Verification items for the finished model (mm, model axes). Face numbers are marked on the shaded views. A direction names the side the tool comes from. Round coordinates to 2 decimals unless told otherwise and drop trailing zeros. Write each loop counter-clockwise with the first axis right and the second up, starting at its lowest first coordinate (ties: lowest second). Pieces come first, ordered by that corner, then holes. Notation, with made-up numbers: (-29.75, 43.25) - (-23.75, 43.25) arc R33 ccw to (-23.75, 73.25) - close; hole circle Ø4 at (-13, 31.25). An arc over 180 degrees is marked (long way). Answer as a JSON object with one key per item and string values.
```python
from build123d import *

# Parameters (mm, degrees)
SCHIZZO2_R               = 4.5
TAGLIO_ESTRUSIONE1_DEPTH = 60.933296255


with BuildPart() as part:
    # Schizzo1 → Rivoluzione1 (revolve)
    with BuildSketch(Plane.XY):
        Polygon((0, 0), (0, 42), (5, 42), (5, 26), (7.5, 26), (7.5, 23.25), (11, 23.25), (11, 26), (13, 26), (13, 20), (5, 20), (5, 0), align=None)
    revolve(axis=Axis((5, 0, 0), (-1, 0, 0)))

    # Schizzo2 → Taglio-Estrusione1 (cut, through all)
    with BuildSketch(Plane(origin=(5, 0, 0), x_dir=(0, 0, -1), z_dir=(1, 0, 0))):
        with Locations(Location((0, 34, 0), (0, 0, 90))):
            Circle(SCHIZZO2_R)
        with Locations(Location((29.444863729, -17, 0), (0, 0, 90))):
            Circle(SCHIZZO2_R)
        with Locations(Location((-29.444863729, -17, 0), (0, 0, 90))):
            Circle(SCHIZZO2_R)
    extrude(amount=-TAGLIO_ESTRUSIONE1_DEPTH, mode=Mode.SUBTRACT)


solid = part.part
```
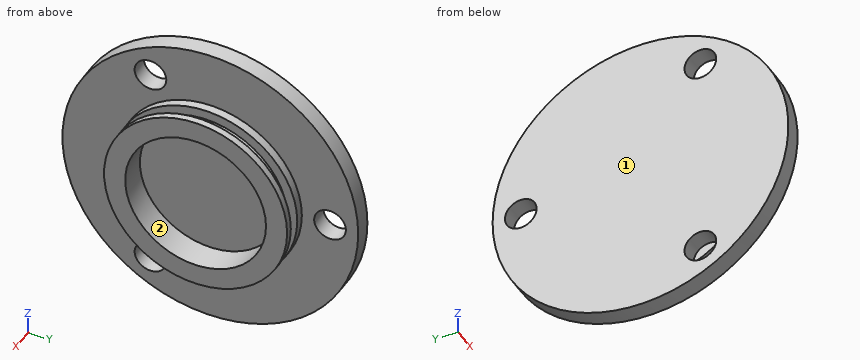
1. Cross-section at B-B (z = 0). Record the boundary of the cut face in (x, y).
Completed:
{"outline": "(0, -42) - (5, -42) - (5, -26) - (7.5, -26) - (7.5, -23.25) - (11, -23.25) - (11, -26) - (13, -26) - (13, -20) - (5, -20) - (5, 20) - (13, 20) - (13, 26) - (11, 26) - (11, 23.25) - (7.5, 23.25) - (7.5, 26) - (5, 26) - (5, 29.5) - (0, 29.5) - close; (0, 38.5) - (5, 38.5) - (5, 42) - (0, 42) - close"}
2. Cross-section at C-C (y = -17). Record the boundary of the cut face in (x, z), plus the area to 3 significant figures.
Completed:
{"outline": "(0, -38.41) - (5, -38.41) - (5, -33.94) - (0, -33.94) - close; (0, -24.94) - (5, -24.94) - (5, -19.67) - (7.5, -19.67) - (7.5, -15.86) - (11, -15.86) - (11, -19.67) - (13, -19.67) - (13, -10.54) - (5, -10.54) - (5, 10.54) - (13, 10.54) - (13, 19.67) - (11, 19.67) - (11, 15.86) - (7.5, 15.86) - (7.5, 19.67) - (5, 19.67) - (5, 24.94) - (0, 24.94) - close; (0, 33.94) - (5, 33.94) - (5, 38.41) - (0, 38.41) - close", "area": "414 mm^2"}
3. Access from +Z, -Z, +X, -X, +Y, -Y to the whole of each face (thin tool, end or side, straight path). Record for the marked faces 1 and 2.
Completed:
{"face 1": "+Z, -Z, -X, +Y, -Y", "face 2": "+X"}
4. Material ranges on probe 1 along Y at (x, z) = (9.75, 0); probe 2 along Z at (x, y) = (2.95, -17), recorded low to high. Write a range as from..to.
Completed:
{"probe 1": "y = -23.25..-20, 20..23.25", "probe 2": "z = -38.41..-33.94, -24.94..24.94, 33.94..38.41"}
5. Cross-section at D-D (x = 12). Record the boundary of the cut face in (y, z).
Completed:
{"outline": "circle Ø52 at (0, 0); hole circle Ø40 at (0, 0)"}
6. Go/stop test with flat-tipped pins: pin 1 (10.5 mm diameter, centred on y = -17, z = 29.44, fed in from +X); pin 2 (5 mm diameter, centred on x = 2, z = -24.5, fed in from -Y); pin 3 (8 mm diameter, centred on y = 34, z = 0, fed in from -X); pin 4 (1.5 mm diameter, centred on x = 11.5, z = 16, fed in from -Y). Record where each tip stops, or that it passes through.
Completed:
{"pin 1": "stops at x = 5", "pin 2": "stops at y = -35.78", "pin 3": "passes through", "pin 4": "stops at y = -21.06"}
7. Cross-section at A-A (y = 34). Record the boundary of the cut face in (x, z), plus the area to 3 significant figures.
Completed:
{"outline": "(0, -24.66) - (5, -24.66) - (5, -4.5) - (0, -4.5) - close; (0, 4.5) - (5, 4.5) - (5, 24.66) - (0, 24.66) - close", "area": "202 mm^2"}
